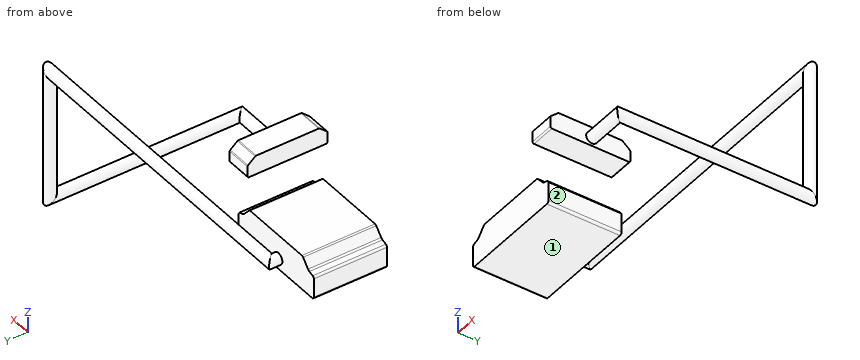
```python
from build123d import *

# Parameters (mm, degrees)
ESQUISSE3_R        = 0.75
BOSS_EXTRU_1_DEPTH = 9.6
BOSS_EXTRU_2_DEPTH = 3.3


with BuildPart() as part:
    # Balayage4: sweep along a curve in space
    with BuildLine() as balayage4_path:
        Line((0, 0, 0), (5, 0, 0))
        Line((5, 0, 0), (5, 25.07, 0))
        Line((5, 25.07, 0), (5, 25.07, 17.06))
        Line((5, 25.07, 17.06), (-35.94, 25.07, 17.06))
        Line((-35.94, 25.07, 17.06), (-35.94, 24.07, 17.06))
    # Esquisse3 → Balayage4 (sweep)
    with BuildSketch(Plane(origin=(0, 0, 0), x_dir=(0, 0, -1), z_dir=(1, 0, 0))):
        Circle(ESQUISSE3_R)
    sweep(path=balayage4_path.line, transition=Transition.RIGHT)

    # Esquisse4 → Boss.-Extru.1 (add)
    with BuildSketch(Plane.XZ.offset(-24.07)):
        with BuildLine():
            Line((-28.529069989, 15.951817831), (-28.529069989, 18.430245431))
            Line((-28.529069989, 18.430245431), (-28.740844235, 18.716979133))
            Line((-28.740844235, 18.716979133), (-29.3555682, 18.906124969))
            Line((-29.3555682, 18.906124969), (-29.606713417, 19.068458081))
            Line((-29.606713417, 19.068458081), (-30.514475757, 20.100006195))
            ThreePointArc((-30.514475757, 20.100006195), (-30.616110911, 20.175182519), (-30.739689812, 20.201817826))
            Line((-30.739689812, 20.201817826), (-40.318450167, 20.201817826))
            Line((-40.318450167, 20.201817826), (-40.543664222, 20.100006195))
            Line((-40.543664222, 20.100006195), (-41.451426562, 19.068458081))
            Line((-41.451426562, 19.068458081), (-41.702571779, 18.906124969))
            Line((-41.702571779, 18.906124969), (-42.317295744, 18.716979133))
            ThreePointArc((-42.317295744, 18.716979133), (-42.470386925, 18.608476003), (-42.529069989, 18.430245431))
            Line((-42.529069989, 18.430245431), (-42.529069989, 15.951817831))
            ThreePointArc((-42.529069989, 15.951817831), (-42.441202024, 15.739685796), (-42.229069989, 15.651817831))
            Line((-42.229069989, 15.651817831), (-28.829069989, 15.651817831))
            ThreePointArc((-28.829069989, 15.651817831), (-28.616937955, 15.739685796), (-28.529069989, 15.951817831))
        make_face()
    extrude(amount=BOSS_EXTRU_1_DEPTH)

    # Esquisse5 → Boss.-Extru.2 (add)
    with BuildSketch(Plane.ZY):
        with BuildLine():
            Line((-1.092354738, 4.837960255), (-1.092354738, -5.262039745))
            ThreePointArc((-1.092354738, -5.262039745), (-1.033776094, -5.403461102), (-0.892354738, -5.462039745))
            Line((-0.892354738, -5.462039745), (0.498872789, -5.443254351))
            Line((0.498872789, -5.443254351), (1.360996797, -4.442758746))
            Line((1.360996797, -4.442758746), (1.407645262, -4.314371414))
            Line((1.407645262, -4.314371414), (1.407645262, 3.890291924))
            Line((1.407645262, 3.890291924), (1.360996797, 4.018679255))
            Line((1.360996797, 4.018679255), (0.567600055, 4.966347586))
            Line((0.567600055, 4.966347586), (0.41424852, 5.037960255))
            Line((0.41424852, 5.037960255), (-0.892354738, 5.037960255))
            ThreePointArc((-0.892354738, 5.037960255), (-1.033776094, 4.979381611), (-1.092354738, 4.837960255))
        make_face()
    extrude(amount=BOSS_EXTRU_2_DEPTH)


solid = part.part
```
Read the model definition and answer for the solid it produces. Units are mm, in the model's axes. Face numbers are marked on the shaded views. A direction names the side the tool comes from. Coordinates: 2 decimals unless noted, no trailing zeros. Loops run counter-clockwise (first coordinate to the right, second up) from the corner with the lowest first, then second, coordinate; pieces in that order, holes last. Notation, with made-up numbers: (10.25, -38.75) -> (31.25, -38.75) arc R19 cw to (31.25, -24.75) -> close; hole circle Ø11 at (50, 39). An arc over 180 degrees is marked (long way). Return JSON: item names as keys, results as strings.
Item 1: Find section B-B (z = 17.06). Determine the outline of the cut face in (x, y).
Answers:
{"outline": "(-42.53, 14.47) -> (-28.53, 14.47) -> (-28.53, 24.07) -> (-35.19, 24.07) -> (-35.19, 24.32) -> (5, 24.32) arc R0.75 ccw to (5, 25.82) -> (-36.69, 25.82) -> (-36.69, 24.07) -> (-42.53, 24.07) -> close"}
Item 2: Find section D-D (x = 2). Determine the outline of the cut face in (y, z), plus the area to 3 significant figures.
Answers:
{"outline": "circle Ø1.5 at (0, 0); circle Ø1.5 at (25.07, 17.06)", "area": "3.53 mm2"}
Item 3: For the marked faces 1 and 2, determine the directions among +Z, -Z, +X, -X, +Y, -Y from which every point of the face is accessible in a straight line to the end or side of a thin tool.
Answers:
{"face 1": "-Z, +X, -X, +Y, -Y", "face 2": "+Z, -Z, +X, -Y"}
Item 4: Find the intervals of material crossed by probe 1 along Z at (x, y) = (-40, 20); probe 2 along Y at (x, z) = (-39.5, 15.75); probe 3 along X at (y, z) = (2.5, 0.5), in increasing order.
Answers:
{"probe 1": "z = 15.65 to 20.2", "probe 2": "y = 14.47 to 24.07", "probe 3": "x = -3.3 to 0, 4.44 to 5.56"}
Item 5: Find section C-C (y = 0). Determine the outline of the cut face in (x, z).
Answers:
{"outline": "(-3.3, -1.09) -> (0, -1.09) -> (0, -0.75) -> (5, -0.75) arc R0.75 ccw to (5, 0.75) -> (0, 0.75) -> (0, 1.41) -> (-3.3, 1.41) -> close"}
Item 6: Flat-ended cylindrical pins translate along their axes: P1, Ø3, axis at y = 0, z = 0.5, coming from the +X side; P2, Ø5, axis at x = -36.5, z = 19, coming from the -Y side; P3, Ø1.6, axis at x = -1.5, y = -2, coming from the +Z side; P4, Ø1.2, axis at y = 19.5, z = 17, coming from the +X side. Find the tip coordinate at first contact, or state that the pin passes through.
Answers:
{"P1": "stops at x = 5.75", "P2": "stops at y = 14.47", "P3": "stops at z = 1.41", "P4": "stops at x = -28.53"}
Item 7: Find section A-A (y = 21). Determine the outline of the cut face in (x, z), plus the area to 3 significant figures.
Answers:
{"outline": "(-42.53, 15.95) arc R0.3 ccw to (-42.23, 15.65) -> (-28.83, 15.65) arc R0.3 ccw to (-28.53, 15.95) -> (-28.53, 18.43) -> (-28.74, 18.72) -> (-29.36, 18.91) -> (-29.61, 19.07) -> (-30.51, 20.1) arc R0.3 ccw to (-30.74, 20.2) -> (-40.32, 20.2) -> (-40.54, 20.1) -> (-41.45, 19.07) -> (-41.7, 18.91) -> (-42.32, 18.72) arc R0.3 ccw to (-42.53, 18.43) -> close; circle Ø1.5 at (5, 0)", "area": "61.3 mm2"}
